Here's the drawing with two shaded views (mm, measured from the low corner). I have some questions. Coordinates: 2 decimals unless noted, no trailing zeros. Loops run counter-clockwise (first coordinate to the right, second up) from the corner with the lowest first, then second, coordinate; pieces in that order, holes last. Notation, with made-up numbers: M 30.25,-16.75 L 41.25,-16.75 A27 cw 41.25,-0.75 Z; hole C 57.5,-29.75 d10. An arc over 180 degrees is marked long. Return JSON: item names as keys, results as strings. Group by question number.
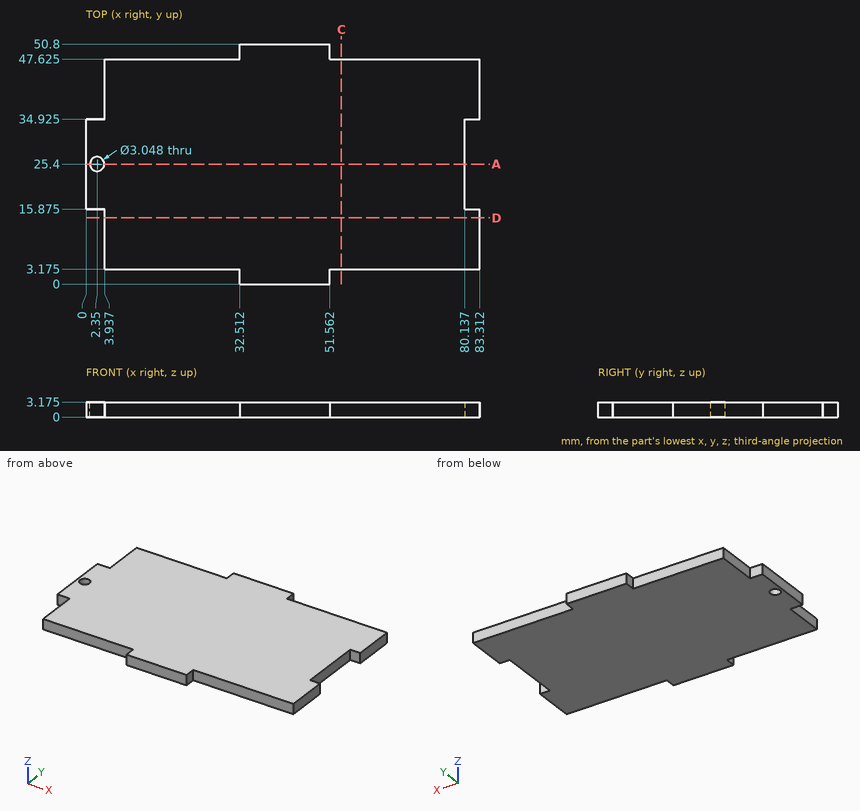
1) For pin 1 (1 mm diameter, centred on x = 61, z = 2.5, fed in from -Y) (1 decimal); pin 2 (1.6 mm diameter, centred on x = 1.5, z = 2, fed in from +Y) (1 decimal); pin 3 (1 mm diameter, centred on x = 69, z = 2, fed in from +Y) (1 decimal), each with a flat end and sliding along its axis, tell me the tip position at first contact or that it passes through.
2) If I drill on line 1 (Y direction, x = 78.5, z = 2) (1 decimal); line 2 (X direction, y = 21.5, z = 1.2); line 3 (X direction, y = 7, z = 2.6), over which ranges is the centre line in solid material (lowest first)? Write a range as from..to.
3) Suppose I cut it at C-C, the plane x = 54. List the corners of the cut face in (y, z) for me (1 decimal), then the cut area to 3 significant figures.
4) Suppose I cut it at A-A, the plane y = 25.4. List the corners of the cut face in (x, z) for me (1 decimal).
5) Suppose I cut it at D-D, the plane y = 14. List the corners of the cut face in (x, z) for me (1 decimal), then the cut area to 3 significant figures.
Returned:
{
 "1": {"pin 1": "stops at y = 3.2", "pin 2": "stops at y = 34.9", "pin 3": "stops at y = 47.6"},
 "2": {"line 1": "y = 3.2..47.6", "line 2": "x = 0..80.14", "line 3": "x = 3.94..83.31"},
 "3": {"outline": "M 3.2,0 L 47.6,0 L 47.6,3.2 L 3.2,3.2 Z", "area": "141 mm²"},
 "4": {"outline": "M 0,0 L 0.8,0 L 0.8,3.2 L 0,3.2 Z; M 3.9,0 L 80.1,0 L 80.1,3.2 L 3.9,3.2 Z"},
 "5": {"outline": "M 3.9,0 L 83.3,0 L 83.3,3.2 L 3.9,3.2 Z", "area": "252 mm²"}
}
